Part model, mm, in its own coordinate system. A direction names the side the tool comes from. Round coordinates to 2 decimals unless told otherwise and drop trailing zeros. Write each loop counter-clockwise with the first axis right and the second up, starting at its lowest first coordinate (ties: lowest second). Pieces come first, ordered by that corner, then holes. Notation, with made-up numbers: (42, -29.75) -> (78, -29.75) arc R19 ccw to (78, -5.75) -> close; hole circle Ø4 at (24, -32). An arc over 180 degrees is marked (long way). Use CSV: the item, a comma, the result in double quotes. Start each with the question number.
(1) Probe line 1 (Y direction, x = 50.5, z = 0); line 2 (Y direction, x = 4.5, z = -13). List the from-to ranges inside material, lowest first. Write a range as [from, to].
(2) Saw through at A-A (z = -12.5). Give the cut face in (x, y) (3 decimals).
(3) Drop flat-ended pins along their axis: pin 1 (1 mm diameter, centred on x = 87, z = 7, fed in from +Y); pin 2 (1.5 mm diameter, centred on y = 47.5, z = -9, fed in from +X); pin 3 (1 mm diameter, centred on x = 11, z = -20, fed in from +Y). Give the stop position or say it passes through.
(4) Saw through at B-B (x = 45). Give the cut face in (y, z).
(5) Which spindle directions (+Z, -Z, +X, -X, +Y, -Y) get a long thin tool onto all of the face, cutting with end or side? Do faces 1 (the flat face through (12.7, 57, -1)), 2 (the flat face through (28, 10, -50)). Say none if no direction does.
Autodesk Inventor part; units mm, degrees
ref_plane "YZ Plane" through (0, 0, 0) normal (1, 0, 0) x (0, 1, 0)
ref_plane "XZ Plane" through (0, 0, 0) normal (0, 1, 0) x (-1, 0, 0)
ref_plane "XY Plane" through (0, 0, 0) normal (0, 0, 1) x (1, 0, 0)
sketch "Sketch1" plane through (0, 0, 0) normal (0, 0, 1) x (1, 0, 0)
  line L0 (0, 0) -> (0, 101.6)
  line L1 (0, 101.6) -> (1.524, 101.6)
  line L2 (12.7, 90.424) -> (12.7, 22.225)
  line L3 (0, 0) -> (101.6, 0)
  line L4 (101.6, 0) -> (101.6, 1.524)
  line L5 (90.424, 12.7) -> (22.225, 12.7)
  arc A0 (12.7, 22.225) -> (22.225, 12.7) centre (22.225, 22.225) ccw
  arc A1 (12.7, 90.424) -> (1.524, 101.6) centre (1.524, 90.424) ccw
  arc A2 (101.6, 1.524) -> (90.424, 12.7) centre (90.424, 1.524) ccw
  dimension "thickness" = 12.7
  dimension "d3" = 12.7
  dimension "LegSize" = 101.6
  dimension "d5" = 101.6
  dimension "radius" = 9.525
  dimension "d7" = 11.176
  dimension "d8" = 11.176
extrude "4\" X 4\" X 1/2\"" add sketch "Sketch1" along normal mid plane 100
equation "\"d3\" = thickness"
equation "\"d5\" = LegSize"
properties part number "ANGLE IRON, 4 X 4 X 0.50 THK" material "Angle Iron"
Answers:
1,line 1,"y = [0, 12.7]"
1,line 2,"y = [0, 101.2]"
2,outline,"(0, 0) -> (101.6, 0) -> (101.6, 1.524) arc R11.176 ccw to (90.424, 12.7) -> (22.225, 12.7) arc R9.525 cw to (12.7, 22.225) -> (12.7, 90.424) arc R11.176 ccw to (1.524, 101.6) -> (0, 101.6) -> close"
3,pin 1,"stops at y = 12.7"
3,pin 2,"stops at x = 12.7"
3,pin 3,"stops at y = 97.08"
4,outline,"(0, -50) -> (12.7, -50) -> (12.7, 50) -> (0, 50) -> close"
5,face 1,"+Z, -Z, +X, +Y"
5,face 2,"-Z, +X, -X, +Y, -Y"
